from build123d import *

# Parameters (mm, degrees)
SKETCH1_W           = 203.2
SKETCH1_H           = 203.2
BOSS_EXTRUDE1_DEPTH = 6.35
SKETCH2_W           = 25.4
SKETCH2_H           = 25.4
SKETCH2_W_2         = 12.7
SKETCH2_H_2         = 12.7
BOSS_EXTRUDE2_DEPTH = 31.75
SKETCH3_R           = 3.906287384
CUT_EXTRUDE1_DEPTH  = 25.4
SKETCH4_R           = 3.81
CUT_EXTRUDE2_DEPTH  = 25.4


with BuildPart() as part:
    # Sketch1 → Boss-Extrude1 (new body)
    with BuildSketch(Plane(origin=(0, 0, 0), x_dir=(1, 0, 0), z_dir=(0, 1, 0))):
        Rectangle(SKETCH1_W, SKETCH1_H)
    extrude(amount=BOSS_EXTRUDE1_DEPTH)

    # Sketch2 → Boss-Extrude2 (add)
    with BuildSketch(Plane(origin=(0, 0, 0), x_dir=(1, 0, 0), z_dir=(0, 1, 0))):
        Rectangle(SKETCH2_W, SKETCH2_H)
        Rectangle(SKETCH2_W_2, SKETCH2_H_2, mode=Mode.SUBTRACT)
    extrude(amount=BOSS_EXTRUDE2_DEPTH)

    # Sketch3 → Cut-Extrude1 (cut)
    with BuildSketch(Plane.XY.offset(12.7)):
        with Locations((0, 19.05)):
            Circle(SKETCH3_R)
    extrude(amount=-CUT_EXTRUDE1_DEPTH, mode=Mode.SUBTRACT)

    # Sketch4 → Cut-Extrude2 (cut)
    with BuildSketch(Plane(origin=(0, 6.35, 0), x_dir=(1, 0, 0), z_dir=(0, 1, 0))):
        with Locations((0, 63.5)):
            Circle(SKETCH4_R)
    extrude(amount=-CUT_EXTRUDE2_DEPTH, mode=Mode.SUBTRACT)


solid = part.part
For this review, take the finished solid that the model builds, in its own axes (mm). A direction names the side the tool comes from. Give positions to 0.01 mm unless a question says otherwise; leave off trailing zeros. Loops run counter-clockwise (first coordinate to the right, second up) from the corner with the lowest first, then second, coordinate; pieces in that order, holes last.
Item 1: Take a section at D-D, the plane z = -20. State the section outline as (x, y) points.
Item 2: Take a section at B-B, the plane z = -63.5. State the section outline as (x, y) points.
Item 3: Take a section at A-A, the plane y = 19.05. State the section outline as (x, z) points.
Item 4: Tool access review of faces 4 (the flat face through (12.7, 19, 0)), 5 (the flat face through (-6.35, 19, 0)), 6 (the flat face through (-12.7, 19, 0)), 7 (the flat face through (-3, 16, -12.7)): name each direction out of +Z, -Z, +X, -X, +Y, -Y from which nothing blocks a thin tool from reaching the whole face with its end or side.
Item 5: Take a section at C-C, the plane x = 0. State the section outline as (y, z) points.
Item 6: Insertion check: pin 1 (6 mm diameter, centred on x = -1, y = 25.5, fed in from +Z); pin 2 (6 mm diameter, centred on x = 60.5, z = -19, fed in from +Y); pin 3 (4 mm diameter, centred on y = 14.5, z = 1.5, fed in from -X). Each pin has a flat end and moves straight along its axis. Give the tip position at first contact, or say it passes through.
Item 7: For line 1 along X through (y, z) = (29.5, -4.5); line 2 along Y through (x, z) = (0, 9), list the stretches that pass through material, from the lowest coordinate up.
Item 8: Draft analysis for pull direction Y (two halves, no side actions). For faces 1 (the cylindrical face through (-0.847, 15.237, 9.569)), 2 (the flat face through (101.6, 3, 1)), 3 (the flat face through (0, 6.35, 0)), state which applies: +Y half, -Y half, draft (parallel to the pull), parting line (faces both ways), or undercut.
Calculated:
1. outline: (-101.6, 0) - (101.6, 0) - (101.6, 6.35) - (-101.6, 6.35) - close
2. outline: (-101.6, 0) - (-3.81, 0) - (-3.81, 6.35) - (-101.6, 6.35) - close; (3.81, 0) - (101.6, 0) - (101.6, 6.35) - (3.81, 6.35) - close
3. outline: (-12.7, -12.7) - (-3.91, -12.7) - (-3.91, -6.35) - (-6.35, -6.35) - (-6.35, 6.35) - (-3.91, 6.35) - (-3.91, 12.7) - (-12.7, 12.7) - close; (3.91, -12.7) - (12.7, -12.7) - (12.7, 12.7) - (3.91, 12.7) - (3.91, 6.35) - (6.35, 6.35) - (6.35, -6.35) - (3.91, -6.35) - close
4. face 4: +Z, -Z, +X, +Y
4. face 5: +Y
4. face 6: +Z, -Z, -X, +Y
4. face 7: -Z, +X, -X, +Y
5. outline: (0, -101.6) - (6.35, -101.6) - (6.35, -67.31) - (0, -67.31) - close; (0, -59.69) - (6.35, -59.69) - (6.35, -12.7) - (15.14, -12.7) - (15.14, -6.35) - (6.35, -6.35) - (6.35, 6.35) - (15.14, 6.35) - (15.14, 12.7) - (6.35, 12.7) - (6.35, 101.6) - (0, 101.6) - close; (22.96, -12.7) - (31.75, -12.7) - (31.75, -6.35) - (22.96, -6.35) - close; (22.96, 6.35) - (31.75, 6.35) - (31.75, 12.7) - (22.96, 12.7) - close
6. pin 1: stops at z = 12.7
6. pin 2: stops at y = 6.35
6. pin 3: stops at x = -12.7
7. line 1: x = -12.7 to -6.35, 6.35 to 12.7
7. line 2: y = 0 to 15.14, 22.96 to 31.75
8. face 1: undercut
8. face 2: draft
8. face 3: +Y half
